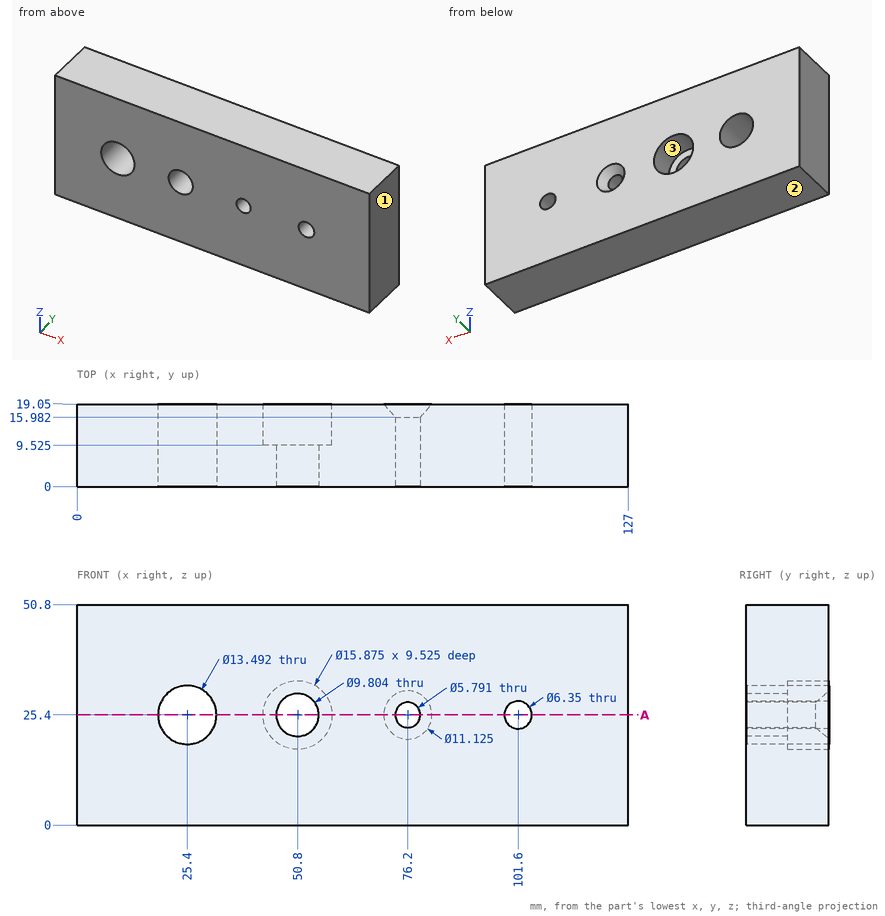
Design review of the part shown in the three views and the two pictorial views. Dimensions are in mm from the part's minimum x, y and z. Round coordinates to 2 decimals unless told otherwise and drop trailing zeros. Write item = value, one per line. Start each with the question number.
1) The part is to be moulded in two halves that separate along Z. For the marked faces 1, 2 and 3, say which applies: +Z half, -Z half, draft (parallel to the pull), parting line (faces both ways), or undercut.
2) Take a section at A-A on z = 25.4. Count the separate pieces of the cut face and the enclosed holes in it, plus the area to 3 significant figures.
3) To check wall thickness, follow line 1 (X direction, y = 3.25, z = 25.4) (1 decimal); line 2 (Z direction, x = 101.6, y = 4.25) (1 decimal); line 3 (Z direction, x = 22.5, y = 14). State the ranges of each line that lie inside material, in increasing order. Write a range as from..to.
4) Insertion check: pin 1 (3.5 mm diameter, centred on x = 76.2, z = 25.4, fed in from +Y); pin 2 (12.5 mm diameter, centred on x = 50.8, z = 25.4, fed in from +Y) (1 decimal). Each pin has a flat end and moves straight along its axis. Give the tip position at first contact, or say it passes through.
Verdict:
q1.face_1 = draft
q1.face_2 = -Z half
q1.face_3 = undercut
q2.separate_pieces = 5
q2.enclosed_holes = 0
q2.area = 1,680 mm2
q3.line_1 = 0..18.7, 32.1..45.9, 55.7..73.3, 79.1..98.4, 104.8..127
q3.line_2 = 0..22.2, 28.6..50.8
q3.line_3 = 0..19.31, 31.49..50.8
q4.pin_1 = through
q4.pin_2 = 9.5
